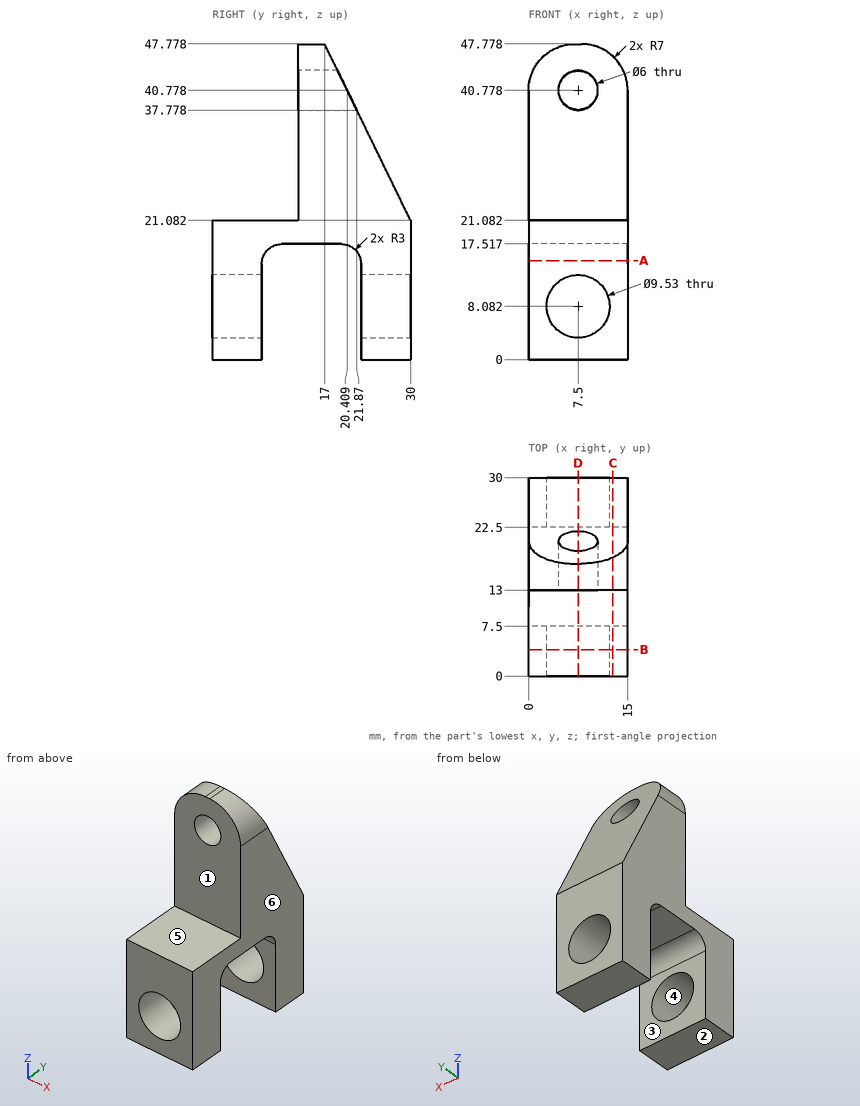
Geometry: see drawing. Coordinates: mm, zero at the bounding-box minimum. A direction names the side the tool comes from. Give positions to 0.01 mm unless a question says otherwise; leave off trailing zeros. Loops run counter-clockwise (first coordinate to the right, second up) from the corner with the lowest first, then second, coordinate; pieces in that order, holes last. Notation, with made-up numbers: (-20, 6) - (-4, 6) arc R24 ccw to (-4, 42) - close; hole circle Ø9 at (37.25, -34.5). An arc over 180 degrees is marked (long way). Use CSV: the item, a comma, the result in double quotes. Start each with the question number.
1. Draft query along X for the marked faces 4, 5 and 6. Return one class per face: +X half, -X half, draft (parallel to the pull), parting line (faces both ways), or undercut.
2. Pin query (flat end, axial travel): pin 1 (7.5 mm diameter, centred on x = 7.5, z = 8.08, fed in from +Y); pin 2 (6.5 mm diameter, centred on x = 5.5, y = 7.5, fed in from +Z); pin 3 (7 mm diameter, centred on x = 6.5, y = 14.5, fed in from -Z); pin 4 (4 mm diameter, centred on x = 4, y = 20, fed in from +Z) (1 decimal). Return the tip coordinate at first contact, or that it passes through.
3. Ray query, L1, parallel to Y at x = 12, z = 2; L2, parallel to X at y = 26, z = 5 (1 decimal); L3, parallel to X at y = 22.75, z = 12 (1 decimal). Return the intervals inside material, ascending.
4. Section B-B (y = 4). Output: boundary loops of the cut face in (x, z) (1 decimal).
5. Reachability of the marked faces 1, 2 and 3 from +Z, -Z, +X, -X, +Y, -Y: full face, straight path, thin tool, end or side. Return the list, or none.
6. Section D-D (x = 7.5). Output: boundary loops of the cut face in (y, z).
7. Section C-C (x = 12.75). Output: boundary loops of the cut face in (y, z) (1 decimal).
8. Section A-A (z = 15). Output: boundary loops of the cut face in (x, y), then the cut area to 3 significant figures.
Response:
1,face 4,"undercut"
1,face 5,"draft"
1,face 6,"+X half"
2,pin 1,"through"
2,pin 2,"z = 21.08"
2,pin 3,"z = 17.52"
2,pin 4,"z = 45.7"
3,L1,"0 to 7.5, 22.5 to 30"
3,L2,"0 to 3.9, 11.1 to 15"
3,L3,"0 to 4.8, 10.2 to 15"
4,outline,"(0, 0) - (15, 0) - (15, 21.1) - (0, 21.1) - close; hole circle Ø9.5 at (7.5, 8.1)"
5,face 1,"+Z, +X, -X, -Y"
5,face 2,"-Z, +X, -X, +Y, -Y"
5,face 3,"-Z, +X, -X"
6,outline,"(0, 0) - (7.5, 0) - (7.5, 3.32) - (0, 3.32) - close; (0, 12.85) - (7.5, 12.85) - (7.5, 14.52) arc R3 cw to (10.5, 17.52) - (19.5, 17.52) arc R3 cw to (22.5, 14.52) - (22.5, 12.85) - (30, 12.85) - (30, 21.08) - (21.87, 37.78) - (13, 37.78) - (13, 21.08) - (0, 21.08) - close; (13, 43.78) - (18.95, 43.78) - (17, 47.78) - (13, 47.78) - close; (22.5, 0) - (30, 0) - (30, 3.32) - (22.5, 3.32) - close"
7,outline,"(0, 0) - (7.5, 0) - (7.5, 14.5) arc R3 cw to (10.5, 17.5) - (19.5, 17.5) arc R3 cw to (22.5, 14.5) - (22.5, 0) - (30, 0) - (30, 21.1) - (17.9, 45.9) - (13, 45.9) - (13, 21.1) - (0, 21.1) - close"
8,outline,"(0, 0) - (15, 0) - (15, 7.54) - (0, 7.54) - close; (0, 22.46) - (15, 22.46) - (15, 30) - (0, 30) - close"
8,area,"226 mm²"
